from build123d import *

# Parameters (mm, degrees)
BOSS_EXTRUDE1_DEPTH = 140
FILLET1_R           = 50
FILLET2_R           = 50
CUT_EXTRUDE1_DEPTH  = 150
SKETCH4_R           = 1.5
CUT_EXTRUDE2_DEPTH  = 10
SKETCH5_R           = 3
SKETCH5_R_2         = 1.5
BOSS_EXTRUDE2_DEPTH = 12


with BuildPart() as part:
    # Sketch1 → Boss-Extrude1 (new body)
    with BuildSketch(Plane.XY):
        Polygon((0, 0), (150, 0), (168.793852416, -6.840402867), (169.819912846, -4.021325004), (150.528980942, 3), (-0.528980942, 3), (-19.819912846, -4.021325004), (-18.793852416, -6.840402867), align=None)
    extrude(amount=BOSS_EXTRUDE1_DEPTH)

    # Fillet1
    fillet1_edges = [part.edges().sort_by_distance(p)[0] for p in [
        (-0.528980942, 3, 70),
        (150.528980942, 3, 70),
    ]]
    fillet(fillet1_edges, radius=FILLET1_R)

    # Fillet2
    fillet2_edges = [part.edges().sort_by_distance(p)[0] for p in [
        (150, 0, 70),
        (0, 0, 70),
    ]]
    fillet(fillet2_edges, radius=FILLET2_R)

    # Sketch3 → Cut-Extrude1 (cut)
    with BuildSketch(Plane(origin=(0, 3, 0), x_dir=(1, 0, 0), z_dir=(0, 1, 0))):
        Polygon((101.712631907, -140), (101.712631907, -130.960680496), (106.212631907, -130.960680496), (106.212631907, -109.960680496), (94.212631907, -109.960680496), (94.212631907, -130.960680496), (98.712631907, -130.960680496), (98.712631907, -140), align=None)
        Polygon((51.287368093, -140), (51.287368093, -130.960680496), (55.787368093, -130.960680496), (55.787368093, -109.960680496), (43.787368093, -109.960680496), (43.787368093, -130.960680496), (48.287368093, -130.960680496), (48.287368093, -140), align=None)
    extrude(amount=-CUT_EXTRUDE1_DEPTH, mode=Mode.SUBTRACT)

    # Sketch4 → Cut-Extrude2 (cut)
    with BuildSketch(Plane(origin=(0, 3, 0), x_dir=(1, 0, 0), z_dir=(0, 1, 0))):
        with Locations(Location((134.997368093, -5, 0), (0, 0, 180))):
            Circle(SKETCH4_R)
        with Locations(Location((14.997368093, -5, 0), (0, 0, 180))):
            Circle(SKETCH4_R)
        with Locations(Location((135.002631907, -64.999999769, 0), (0, 0, 180))):
            Circle(SKETCH4_R)
        with Locations(Location((14.997368093, -64.999999769, 0), (0, 0, 180))):
            Circle(SKETCH4_R)
    extrude(amount=-CUT_EXTRUDE2_DEPTH, mode=Mode.SUBTRACT)

    # Sketch5 → Boss-Extrude2 (add)
    # profile 1 of 4: a face of its own
    with BuildSketch(Plane(origin=(0, 3, 0), x_dir=(1, 0, 0), z_dir=(0, 1, 0))):
        with Locations(Location((14.997368093, -5, 0), (0, 0, 180))):
            Circle(SKETCH5_R)
        with Locations(Location((14.997368093, -5, 0), (0, 0, 180))):
            Circle(SKETCH5_R_2, mode=Mode.SUBTRACT)
    # profile 2 of 4: a face of its own
    with BuildSketch(Plane(origin=(0, 3, 0), x_dir=(1, 0, 0), z_dir=(0, 1, 0))):
        with Locations(Location((134.997368093, -5, 0), (0, 0, 180))):
            Circle(SKETCH5_R)
        with Locations(Location((134.997368093, -5, 0), (0, 0, 180))):
            Circle(SKETCH5_R_2, mode=Mode.SUBTRACT)
    # profile 3 of 4: a face of its own
    with BuildSketch(Plane(origin=(0, 3, 0), x_dir=(1, 0, 0), z_dir=(0, 1, 0))):
        with Locations(Location((135.002631907, -64.999999769, 0), (0, 0, 180))):
            Circle(SKETCH5_R)
        with Locations(Location((135.002631907, -64.999999769, 0), (0, 0, 180))):
            Circle(SKETCH5_R_2, mode=Mode.SUBTRACT)
    # profile 4 of 4: a face of its own
    with BuildSketch(Plane(origin=(0, 3, 0), x_dir=(1, 0, 0), z_dir=(0, 1, 0))):
        with Locations(Location((14.997368093, -64.999999769, 0), (0, 0, 180))):
            Circle(SKETCH5_R)
        with Locations(Location((14.997368093, -64.999999769, 0), (0, 0, 180))):
            Circle(SKETCH5_R_2, mode=Mode.SUBTRACT)
    extrude(amount=-BOSS_EXTRUDE2_DEPTH)


solid = part.part
Work out the finished part from the listing and answer in its coordinate system (mm). A direction names the side the tool comes from. Round coordinates to 2 decimals unless told otherwise and drop trailing zeros. Write each loop counter-clockwise with the first axis right and the second up, starting at its lowest first coordinate (ties: lowest second). Pieces come first, ordered by that corner, then holes.
1) A cutting plane is placed at C-C (x = 74). Give the vertices of the cut face in (y, z).
2) A cutting plane is placed at B-B (z = 77.5). Give the vertices of the cut face in (x, y), plus the area to 3 significant figures.
3) A tool of negligible diameter and unlimited length cuts with its end or side. For faces 1 (the flat face through (14, 1, 140)), 2 (the flat face through (-13.613, -4.955, 69.02)), 3 (the cylindrical face through (137.994, -4.437, 5.132)), from which of +Z, -Z, +X, -X, +Y, -Y can it reach the whole face along a straight path? Write none if from no direction.
4) Straight lines are drawn through the part: line 1 (Y direction, x = 128.5, z = 94); line 2 (Z direction, x = 133, y = -3.25); line 3 (Y direction, x = 156.5, z = 80.5). For each, find the intervals that lie inside material, in ascending order.
5) Given pin 1 Ø1.5 at (x, y) = (136.5, -3) entering from -Z; pin 2 Ø8 at (x, z) = (72.5, 118.5) entering from -Y; pin 3 Ø2.5 at (x, z) = (135, 65) entering from -Y, each flat-ended and moving along its own axis, determine where each tip first touches the part or whether it passes through.
6) A cutting plane is placed at A-A (z = 123). Give the vertices of the cut face in (x, y).
7) The mould has two halves that part along X. Classify faces 4 (the flat face through (133.7, -9, 63.7)), 5 (the flat face through (164.394, -2.046, 69.02)), 6 (the cylindrical face through (133.618, -4.437, 62.338)): pulls with the +X half, pulls with the -X half, needs draft (parallel to the pull), parting line crosses it, or undercut.
Completed:
1. outline: (0, 0) - (3, 0) - (3, 140) - (0, 140) - close
2. outline: (-19.82, -4.02) - (-18.79, -6.84) - (-8.28, -3.02) arc R50 cw to (8.82, 0) - (141.18, 0) arc R50 cw to (158.28, -3.02) - (168.79, -6.84) - (169.82, -4.02) - (158.81, -0.02) arc R50 ccw to (141.71, 3) - (8.29, 3) arc R50 ccw to (-8.81, -0.02) - close
2. area: 573 mm2
3. face 1: +Z, +X, -X, +Y, -Y
3. face 2: +Z, -Z, -Y
3. face 3: -Y
4. line 1: y = 0 to 3
4. line 2: z = 2.76 to 7.24, 62.77 to 67.23
4. line 3: y = -2.4 to 0.76
5. pin 1: stops at z = 2.1
5. pin 2: stops at y = 0
5. pin 3: passes through
6. outline: (-19.82, -4.02) - (-18.79, -6.84) - (-8.28, -3.02) arc R50 cw to (8.82, 0) - (43.79, 0) - (43.79, 3) - (8.29, 3) arc R50 ccw to (-8.81, -0.02) - close; (55.79, 0) - (94.21, 0) - (94.21, 3) - (55.79, 3) - close; (106.21, 0) - (141.18, 0) arc R50 cw to (158.28, -3.02) - (168.79, -6.84) - (169.82, -4.02) - (158.81, -0.02) arc R50 ccw to (141.71, 3) - (106.21, 3) - close
7. face 4: needs draft
7. face 5: pulls with the +X half
7. face 6: undercut
